```python
from build123d import *

# Parameters (mm, degrees)
F0_R     = 4.5
F0_W     = 8
F0_H     = 34
F1_DEPTH = 1.2
F2_W     = 4.8
F2_H     = 56
F3_DEPTH = 25
F5_W     = 101.632081
F5_H     = 108.945377
F6_DEPTH = 50


with BuildPart() as f1:
    # F0 (on Top) → F1 (new body)
    with BuildSketch(Plane.XY):
        with BuildLine():
            Line((17.75, 17), (17.75, 30))
            Line((17.75, 30), (-17.75, 30))
            Line((-17.75, 30), (-17.75, 17))
            Line((-17.75, 17), (-9.75, 17))
            Line((-9.75, 17), (-9.75, 17.5))
            ThreePointArc((-9.75, 17.5), (-8.431981, 20.681981), (-5.25, 22))
            Line((-5.25, 22), (5.25, 22))
            ThreePointArc((5.25, 22), (8.431981, 20.681981), (9.75, 17.5))
            Line((9.75, 17.5), (9.75, 17))
            Line((9.75, 17), (17.75, 17))
        make_face()
        with BuildLine():
            Line((28, 30), (17.75, 30))
            Line((17.75, 30), (17.75, 17))
            Line((17.75, 17), (28, 17))
            ThreePointArc((28, 17), (31.181981, 18.318019), (32.5, 21.5))
            Line((32.5, 21.5), (32.5, 25.5))
            ThreePointArc((32.5, 25.5), (31.181981, 28.681981), (28, 30))
        make_face()
        with Locations((25, 23.5)):
            Circle(F0_R, mode=Mode.SUBTRACT)
        with BuildLine():
            Line((-17.75, 17), (-17.75, 30))
            Line((-17.75, 30), (-28, 30))
            ThreePointArc((-28, 30), (-31.181981, 28.681981), (-32.5, 25.5))
            Line((-32.5, 25.5), (-32.5, 21.5))
            ThreePointArc((-32.5, 21.5), (-31.181981, 18.318019), (-28, 17))
            Line((-28, 17), (-17.75, 17))
        make_face()
        with Locations((-25, 23.5)):
            Circle(F0_R, mode=Mode.SUBTRACT)
        with Locations((13.75, 0)):
            Rectangle(F0_W, F0_H)
        with Locations((-13.75, 0)):
            Rectangle(F0_W, F0_H)
        with BuildLine():
            Line((28, -17), (17.75, -17))
            Line((17.75, -17), (17.75, -30))
            Line((17.75, -30), (28, -30))
            ThreePointArc((28, -30), (31.181981, -28.681981), (32.5, -25.5))
            Line((32.5, -25.5), (32.5, -21.5))
            ThreePointArc((32.5, -21.5), (31.181981, -18.318019), (28, -17))
        make_face()
        with Locations((25, -23.5)):
            Circle(F0_R, mode=Mode.SUBTRACT)
        with BuildLine():
            Line((17.75, -30), (17.75, -17))
            Line((17.75, -17), (9.75, -17))
            Line((9.75, -17), (9.75, -17.5))
            ThreePointArc((9.75, -17.5), (8.431981, -20.681981), (5.25, -22))
            Line((5.25, -22), (-5.25, -22))
            ThreePointArc((-5.25, -22), (-8.431981, -20.681981), (-9.75, -17.5))
            Line((-9.75, -17.5), (-9.75, -17))
            Line((-9.75, -17), (-17.75, -17))
            Line((-17.75, -17), (-17.75, -30))
            Line((-17.75, -30), (17.75, -30))
        make_face()
        with BuildLine():
            Line((-17.75, -30), (-17.75, -17))
            Line((-17.75, -17), (-28, -17))
            ThreePointArc((-28, -17), (-31.181981, -18.318019), (-32.5, -21.5))
            Line((-32.5, -21.5), (-32.5, -25.5))
            ThreePointArc((-32.5, -25.5), (-31.181981, -28.681981), (-28, -30))
            Line((-28, -30), (-17.75, -30))
        make_face()
        with Locations((-25, -23.5)):
            Circle(F0_R, mode=Mode.SUBTRACT)
    extrude(amount=F1_DEPTH)

    # F2 (on face) → F3 (join)
    with BuildSketch(Plane.XY.offset(1.2)):
        with Locations((14.15, 0)):
            Rectangle(F2_W, F2_H)
        with Locations((-14.15, 0)):
            Rectangle(F2_W, F2_H)
    extrude(amount=F3_DEPTH)

    # F5 (on face) → F6 (cut)
    with BuildSketch(Plane(origin=(0, -3.217416, 9.902189), x_dir=(1, 0, 0), z_dir=(0, -0.309017, 0.951057))):
        with Locations((3.367923, -6.511665)):
            Rectangle(F5_W, F5_H)
    extrude(amount=F6_DEPTH, mode=Mode.SUBTRACT)


solid = f1.part
```
CAD build for the part. Positions are in the model's coordinates, mm. A direction names the side the tool comes from. Round coordinates to 2 decimals unless told otherwise and drop trailing zeros. Loops run counter-clockwise (first coordinate to the right, second up) from the corner with the lowest first, then second, coordinate; pieces in that order, holes last. Notation, with made-up numbers: M 1.5,86.25 L 43.5,86.25 A27 ccw 43.5,108.25 Z; hole C -12.75,82 d2. An arc over 180 degrees is marked long. Return JSON: item names as keys, results as strings. Group by question number.
(1) Saw through at B-B, the plane y = 4.5. List the corners of the cut face in (x, z), and give its area (3 significant figures).
(2) Saw through at C-C, the plane z = 17. List the corners of the cut face in (x, y).
(3) Drop flat-ended pins along their axis: P1, Ø8, axis at x = -9, z = 10.5, coming from the +Y side; P2, Ø8, axis at x = -25, y = -23.5, coming from the +Z side; P3, Ø1.3, axis at y = 5, z = 0.5, coming from the -X side; P4, Ø1.3, axis at y = -4, z = 0.5, coming from the +X side. Give the stop position or say it passes through.
(4) Mould opens along Y. For faces 1 (the flat face through (14, 28, 10)), 2 (the cylindrical face through (-8.467, 20.647, 0.592)), 3 (the flat face through (-16.55, 6, 8)) say: +Y half, -Y half, draft (parallel to the pull), parting line (faces both ways), or undercut.
(5) Saw through at D-D, the plane y = 23.5. List the corners of the cut face in (x, z), and give its area (3 significant figures).
(6) Tool access for faces 4 (the cylindrical face through (-8.397, -20.717, 0.592)), 5 (the cylindrical face through (31.217, -18.353, 0.592)), 6 (the flat face through (-11.75, 6, 8)), 7 (the cylindrical face through (-31.147, -18.283, 0.592)): list every direction of +Z, -Z, +X, -X, +Y, -Y with a clear straight run to the whole face (end or side of a thin tool).
(7) Saw through at A-A, the plane x = 25. List the corners of the cut face in (y, z).
(8) Wall check: probe 1 along Y at (x, z) = (25, 0.85); probe 2 along X at (y, z) = (2, 5.25); probe 3 along Z at (x, y) = (-10, -6.5). Give the ranges that are in metal, low to high. Write a range as [from, to].
Answer list:
{
 "1": {"outline": "M -17.75,0 L -9.75,0 L -9.75,1.2 L -11.75,1.2 L -11.75,12.41 L -16.55,12.41 L -16.55,1.2 L -17.75,1.2 Z; M 9.75,0 L 17.75,0 L 17.75,1.2 L 16.55,1.2 L 16.55,12.41 L 11.75,12.41 L 11.75,1.2 L 9.75,1.2 Z", "area": "127 mm2"},
 "2": {"outline": "M -16.55,18.63 L -11.75,18.63 L -11.75,28 L -16.55,28 Z; M 11.75,18.63 L 16.55,18.63 L 16.55,28 L 11.75,28 Z"},
 "3": {"P1": "y = 28", "P2": "through", "P3": "x = -17.75", "P4": "x = 17.75"},
 "4": {"face 1": "+Y half", "face 2": "undercut", "face 3": "draft"},
 "5": {"outline": "M -32.5,0 L -29.5,0 L -29.5,1.2 L -32.5,1.2 Z; M -20.5,0 L 20.5,0 L 20.5,1.2 L 16.55,1.2 L 16.55,18.58 L 11.75,18.58 L 11.75,1.2 L -11.75,1.2 L -11.75,18.58 L -16.55,18.58 L -16.55,1.2 L -20.5,1.2 Z; M 29.5,0 L 32.5,0 L 32.5,1.2 L 29.5,1.2 Z", "area": "223 mm2"},
 "6": {"face 4": "+Z, -Z", "face 5": "+Z, -Z, +X", "face 6": "+Z, +Y, -Y", "face 7": "+Z, -Z, -X"},
 "7": {"outline": "M -30,0 L -28,0 L -28,1.2 L -30,1.2 Z; M -19,0 L -17,0 L -17,1.2 L -19,1.2 Z; M 17,0 L 19,0 L 19,1.2 L 17,1.2 Z; M 28,0 L 30,0 L 30,1.2 L 28,1.2 Z"},
 "8": {"probe 1": "[-30, -28], [-19, -17], [17, 19], [28, 30]", "probe 2": "[-16.55, -11.75], [11.75, 16.55]", "probe 3": "[0, 1.2]"}
}
